from build123d import *

# Parameters (mm, degrees)
SKETCH1_R           = 2
BOSS_EXTRUDE1_DEPTH = 3.5
SKETCH2_R           = 0.42
CUT_EXTRUDE1_DEPTH  = 2.5
BOSS_EXTRUDE2_DEPTH = 25.5
BOSS_EXTRUDE3_DEPTH = 25.5


# Read off the part's stored shape, not the designer's step: Boss-Extrude2
with BuildPart() as part:
    # Sketch1 → Boss-Extrude1 (new body)
    with BuildSketch(Plane(origin=(0, 0, 0), x_dir=(1, 0, 0), z_dir=(0, 1, 0))):
        with Locations(Location((0, 0, 0), (0, 0, 270))):
            Circle(SKETCH1_R)
    extrude(amount=BOSS_EXTRUDE1_DEPTH)

    # Sketch2 → Cut-Extrude1 (cut)
    with BuildSketch(Plane(origin=(0, 0, 0), x_dir=(1, 0, 0), z_dir=(0, 1, 0))):
        with Locations(Location((0, 0, 0), (0, 0, 270))):
            Circle(SKETCH2_R)
    extrude(amount=CUT_EXTRUDE1_DEPTH, mode=Mode.SUBTRACT)

    # Boss-Extrude2 outline → Boss-Extrude2 (add)
    with BuildSketch(Plane(origin=(0, 0, 0), x_dir=(0, 0, -1), z_dir=(1, 0, 0))):
        Polygon((-0.42, 1.741182904), (0.42, 0.770925972), (1.072852444, 0.016837151), (1.627531183, 0), (0.42, 1.394780358), (-0.42, 2.36503729), (-1.283933552, 3.362939097), (-1.838612291, 3.379776249), align=None)
    extrude(amount=BOSS_EXTRUDE2_DEPTH)

    # Sketch4 → Boss-Extrude3 (add)
    with BuildSketch(Plane.ZY):
        Polygon((1.627531183, 0), (-1.283933552, 3.362939097), (-1.838612291, 3.379776249), (1.072852444, 0.016837151), align=None)
    extrude(amount=BOSS_EXTRUDE3_DEPTH)


solid = part.part
Build history of the part. All positions in model axes, mm. A direction names the side the tool comes from. Give positions to 0.01 mm unless a question says otherwise; leave off trailing zeros. Order: outer loops, then holes, each group sorted by start corner. A loop starts at its lowest first (then second) coordinate and runs counter-clockwise, first axis right, second up. Notation, with made-up numbers: M 7.5,83 L 57.5,83 A31 cw 57.5,112 Z; hole C 35,-4.5 d2. An arc over 180 degrees is marked long. Put each result on its own line as item: value.
Item 1: Cut at A-A on x = -4. Write the cut outline in (y, z).
Results are:
outline: M 0,1.63 L 0.02,1.07 L 3.38,-1.84 L 3.36,-1.28 Z
Item 2: Pull direction X, two halves, no side cores. Call faces 3 (the face through (25.5, 1.7, 0.1)), 4 (the face through (-0.26, 1.23, -0.33)), 5 (the face through (-13.16, 1.66, 0.19)): +X half, -X half, draft (parallel to the pull), parting line (faces both ways), or undercut.
Results are:
face 3: +X half
face 4: undercut
face 5: draft
Item 3: Drop a flat-ended pin along its axis: pin 1 Ø1.5 at (x, y) = (9.5, 1) entering from -Z. Give the stop position or say it passes through.
Results are:
pin 1: z = -1.41
Item 4: Which spindle directions (+Z, -Z, +X, -X, +Y, -Y) get a long thin tool onto all of the face, cutting with end or side? Do faces 1 (the face through (0, 3.5, 0)), 2 (the face through (-1.774, 1.725, 0.923)). Say none if no direction does.
Results are:
face 1: +Z, -Z, +X, -X, +Y
face 2: none
Item 5: Wall check: probe 1 along X at (y, z) = (0.85, 0); probe 2 along X at (y, z) = (1.25, 0.1). Give the ranges that are in metal, low to high.
Results are:
probe 1: -2 to -0.42, 0.42 to 2
probe 2: -25.5 to 0, 0.41 to 2
